from build123d import *

# Parameters (mm, degrees)
SKETCH2_R          = 7.25
CUT_EXTRUDE1_DEPTH = 10.185586535
SKETCH3_R          = 3.175
CUT_EXTRUDE3_DEPTH = 2.8
SKETCH4_R          = 0.75
CUT_EXTRUDE4_DEPTH = 10.652947736


with BuildPart() as part:
    # Sketch1 → Revolve1 (revolve)
    with BuildSketch(Plane.XY, mode=Mode.PRIVATE) as revolve1_sk:
        Polygon((0, 3.88), (0, 0), (1.67, 0), (1.67, 0.3), (5.075, 0.3), (5.075, 0), (6.25, 0), (6.25, 1.38), (5.075, 1.38), (5.075, 1.08), (2.675, 1.08), (2.675, 3.88), align=None)
    revolve(revolve1_sk.sketch.rotate(Axis((0, 3.88, 0), (0, -1, 0)), 90), axis=Axis((0, 3.88, 0), (0, -1, 0)))

    # Sketch2 → Cut-Extrude1 (cut, through all)
    with BuildSketch(Plane(origin=(0, 1.38, 0), x_dir=(1, 0, 0), z_dir=(0, 1, 0))):
        Circle(SKETCH2_R)
        Polygon((-0.376067993, 5.737688809), (0, 6.25), (0.376067993, 5.737688809), (0.815788701, 6.196530384), (1.121769352, 5.639515362), (1.617619032, 6.037036414), (1.848276925, 5.444848245), (2.391771452, 5.774247078), (2.543159969, 5.157018264), (3.125, 5.412658774), (3.19452884, 4.780950271), (3.804758931, 4.958458377), (3.791238437, 4.323078893), (4.419417382, 4.419417382), (4.323078893, 3.791238437), (4.958458377, 3.804758931), (4.780950271, 3.19452884), (5.412658774, 3.125), (5.157018264, 2.543159969), (5.774247078, 2.391771452), (5.444848245, 1.848276925), (6.037036414, 1.617619032), (5.639515362, 1.121769352), (6.196530384, 0.815788701), (5.737688809, 0.376067993), (6.25, 0), (5.737688809, -0.376067993), (6.196530384, -0.815788701), (5.639515362, -1.121769352), (6.037036414, -1.617619032), (5.444848245, -1.848276925), (5.774247078, -2.391771452), (5.157018264, -2.543159969), (5.412658774, -3.125), (4.780950271, -3.19452884), (4.958458377, -3.804758931), (4.323078893, -3.791238437), (4.419417382, -4.419417382), (3.791238437, -4.323078893), (3.804758931, -4.958458377), (3.19452884, -4.780950271), (3.125, -5.412658774), (2.543159969, -5.157018264), (2.391771452, -5.774247078), (1.848276925, -5.444848245), (1.617619032, -6.037036414), (1.121769352, -5.639515362), (0.815788701, -6.196530384), (0.376067993, -5.737688809), (0, -6.25), (-0.376067993, -5.737688809), (-0.815788701, -6.196530384), (-1.121769352, -5.639515362), (-1.617619032, -6.037036414), (-1.848276925, -5.444848245), (-2.391771452, -5.774247078), (-2.543159969, -5.157018264), (-3.125, -5.412658774), (-3.19452884, -4.780950271), (-3.804758931, -4.958458377), (-3.791238437, -4.323078893), (-4.419417382, -4.419417382), (-4.323078893, -3.791238437), (-4.958458377, -3.804758931), (-4.780950271, -3.19452884), (-5.412658774, -3.125), (-5.157018264, -2.543159969), (-5.774247078, -2.391771452), (-5.444848245, -1.848276925), (-6.037036414, -1.617619032), (-5.639515362, -1.121769352), (-6.196530384, -0.815788701), (-5.737688809, -0.376067993), (-6.25, 0), (-5.737688809, 0.376067993), (-6.196530384, 0.815788701), (-5.639515362, 1.121769352), (-6.037036414, 1.617619032), (-5.444848245, 1.848276925), (-5.774247078, 2.391771452), (-5.157018264, 2.543159969), (-5.412658774, 3.125), (-4.780950271, 3.19452884), (-4.958458377, 3.804758931), (-4.323078893, 3.791238437), (-4.419417382, 4.419417382), (-3.791238437, 4.323078893), (-3.804758931, 4.958458377), (-3.19452884, 4.780950271), (-3.125, 5.412658774), (-2.543159969, 5.157018264), (-2.391771452, 5.774247078), (-1.848276925, 5.444848245), (-1.617619032, 6.037036414), (-1.121769352, 5.639515362), (-0.815788701, 6.196530384), align=None, mode=Mode.SUBTRACT)
    extrude(amount=-CUT_EXTRUDE1_DEPTH, mode=Mode.SUBTRACT)

    # Sketch3 → Cut-Extrude3 (cut)
    with BuildSketch(Plane(origin=(0, 3.88, 0), x_dir=(1, 0, 0), z_dir=(0, 1, 0))):
        Circle(SKETCH3_R)
        Polygon((0, 2.675), (-0.405427797, 1.907387821), (-1.08802052, 2.443734099), (-1.146181242, 1.577583139), (-1.987912408, 1.789924372), (-1.688749537, 0.975), (-2.544076181, 0.82662046), (-1.939317696, 0.203830503), (-2.66034607, -0.279613639), (-1.854560207, -0.602583139), (-2.316617955, -1.3375), (-1.44913241, -1.304804682), (-1.57232555, -2.16412046), (-0.793136454, -1.781413642), (-0.556163773, -2.616544832), (0, -1.95), (0.556163773, -2.616544832), (0.793136454, -1.781413642), (1.57232555, -2.16412046), (1.44913241, -1.304804682), (2.316617955, -1.3375), (1.854560207, -0.602583139), (2.66034607, -0.279613639), (1.939317696, 0.203830503), (2.544076181, 0.82662046), (1.688749537, 0.975), (1.987912408, 1.789924372), (1.146181242, 1.577583139), (1.08802052, 2.443734099), (0.405427797, 1.907387821), align=None, mode=Mode.SUBTRACT)
    extrude(amount=-CUT_EXTRUDE3_DEPTH, mode=Mode.SUBTRACT)

    # Sketch4 → Cut-Extrude4 (cut, through all)
    with BuildSketch(Plane(origin=(0, 3.88, 0), x_dir=(1, 0, 0), z_dir=(0, 1, 0))):
        with Locations(Location((0, 0, 0), (0, 0, 270))):
            Circle(SKETCH4_R)
    extrude(amount=-CUT_EXTRUDE4_DEPTH, mode=Mode.SUBTRACT)


solid = part.part
The listing builds one solid part. Answer for the finished solid, in the listing's coordinates (mm). A direction names the side the tool comes from. Give positions to 0.01 mm unless a question says otherwise; leave off trailing zeros. Write each loop counter-clockwise with the first axis right and the second up, starting at its lowest first coordinate (ties: lowest second). Pieces come first, ordered by that corner, then holes.
1) For a pull along Z with two mould halves and no side action, classify faces 1 (the face through (-1.84, 2.5, -1.39)), 2 (the face through (-2, 1.38, -5)), 3 (the face through (0.225, 1.967, 0.715)) as pulls with the +Z half, pulls with the -Z half, needs draft (parallel to the pull), parting line crosses it, or undercut.
2) Section A-A (x = 3.5) is taken. Write down the section's boundary in (y, z) (3 decimals), and give its area (3 significant figures).
3) Find the intervals of material crossed by L1, parallel to X at y = 1.1, z = -5.25; L2, parallel to Y at x = -3.5, z = -1; L3, parallel to Z at x = -0.25, y = 3.6, in increasing order.
4) Given P1, Ø1, axis at x = 5, y = 2.5, coming from the +Z side; P2, Ø4, axis at x = -4, z = -4.5, coming from the +Y side, each flat-ended and moving along its own axis, determine where each tip first touches the part or whether it passes through.
5) A tool of negligible diameter and unlimited length cuts with its end or side. For faces 4 (the face through (-2, 0, 5)), 5 (the face through (1.88, 2.5, 1.32)), from which of +Z, -Z, +X, -X, +Y, -Y can it reach the whole face along a straight path? Write none if from no direction.
Response:
1. face 1: undercut
1. face 2: needs draft
1. face 3: undercut
2. outline: (0, -4.87) - (1.38, -4.87) - (1.38, -3.675) - (1.08, -3.675) - (1.08, 3.675) - (1.38, 3.675) - (1.38, 4.87) - (0, 4.87) - (0, 3.675) - (0.3, 3.675) - (0.3, -3.675) - (0, -3.675) - close
2. area: 9.03 mm2
3. L1: x = -3.14 to -2.75, -2.52 to 2.52, 2.75 to 3.14
3. L2: y = 0.3 to 1.08
3. L3: z = -2.2 to -0.71, 0.71 to 2.25
4. P1: passes through
4. P2: stops at y = 1.38
5. face 4: +Z, -Z, +X, -X, -Y
5. face 5: +Y
